Input: part model. Units: mm. Frame: model coordinates. Round coordinates to 2 decimals unless told otherwise and drop trailing zeros. Write each loop counter-clockwise with the first axis right and the second up, starting at its lowest first coordinate (ties: lowest second). Pieces come first, ordered by that corner, then holes. Notation, with made-up numbers: (-35.5, -15) - (-10.5, -15) arc R9 ccw to (-10.5, -7) - close; hole circle Ø6 at (46, 11.25). An arc over 180 degrees is marked (long way). Use one line per item in the form item = value.
```python
from build123d import *

# Parameters (mm, degrees)
SKETCH_1_W          = 101
SKETCH_1_H          = 19
SKETCH_1_R          = 2.025
EXTRUDE_1_DEPTH     = 2
CUT_EXTRUDE_1_DEPTH = 2
FILLET_1_R          = 1
FILLET_2_R          = 1


with BuildPart() as part:
    # 草图1 → 凸台-拉伸1 (new body)
    with BuildSketch(Plane.XY):
        Rectangle(SKETCH_1_W, SKETCH_1_H)
        with Locations((-46, 5)):
            Circle(SKETCH_1_R, mode=Mode.SUBTRACT)
        with Locations((46, 5)):
            Circle(SKETCH_1_R, mode=Mode.SUBTRACT)
        with Locations((46, -5)):
            Circle(SKETCH_1_R, mode=Mode.SUBTRACT)
        with Locations((-46, -5)):
            Circle(SKETCH_1_R, mode=Mode.SUBTRACT)
    extrude(amount=EXTRUDE_1_DEPTH)

    # 草图2 → 切除-拉伸1 (cut)
    with BuildSketch(Plane.XY.offset(2)):
        Polygon((-42, 6.5), (-42, -6.5), (-29, 6.5), align=None)
        Polygon((-24.050252532, 6.5), (-37.050252532, -6.5), (-24.050252532, -6.5), align=None)
        Polygon((-2.5, -6.5), (-2.5, 6.5), (-15.5, -6.5), align=None)
        Polygon((-7.449747468, 6.5), (-20.449747468, 6.5), (-20.449747468, -6.5), align=None)
        Polygon((42, -6.5), (29, 6.5), (42, 6.5), align=None)
        Polygon((37.050252532, -6.5), (24.050252532, -6.5), (24.050252532, 6.5), align=None)
        Polygon((20.449747468, -6.5), (7.449747468, 6.5), (20.449747468, 6.5), align=None)
        Polygon((15.5, -6.5), (2.5, -6.5), (2.5, 6.5), align=None)
    extrude(amount=-CUT_EXTRUDE_1_DEPTH, mode=Mode.SUBTRACT)

    # 圆角1
    fillet_1_edges = [part.edges().sort_by_distance(p)[0] for p in [
        (-20.449747468, -6.5, 1),
        (-20.449747468, 6.5, 1),
        (-7.449747468, 6.5, 1),
        (-15.5, -6.5, 1),
        (-2.5, 6.5, 1),
        (-2.5, -6.5, 1),
        (42, 6.5, 1),
        (42, -6.5, 1),
        (29, 6.5, 1),
        (-24.050252532, 6.5, 1),
        (-24.050252532, -6.5, 1),
        (-37.050252532, -6.5, 1),
        (2.5, 6.5, 1),
        (15.5, -6.5, 1),
        (2.5, -6.5, 1),
        (20.449747468, 6.5, 1),
        (20.449747468, -6.5, 1),
        (7.449747468, 6.5, 1),
        (24.050252532, 6.5, 1),
        (37.050252532, -6.5, 1),
        (24.050252532, -6.5, 1),
        (-42, 6.5, 1),
        (-29, 6.5, 1),
        (-42, -6.5, 1),
    ]]
    fillet(fillet_1_edges, radius=FILLET_1_R)

    # 圆角2
    fillet_2_edges = [part.edges().sort_by_distance(p)[0] for p in [
        (-50.5, 9.5, 1),
        (50.5, 9.5, 1),
        (50.5, -9.5, 1),
        (-50.5, -9.5, 1),
    ]]
    fillet(fillet_2_edges, radius=FILLET_2_R)


solid = part.part
```
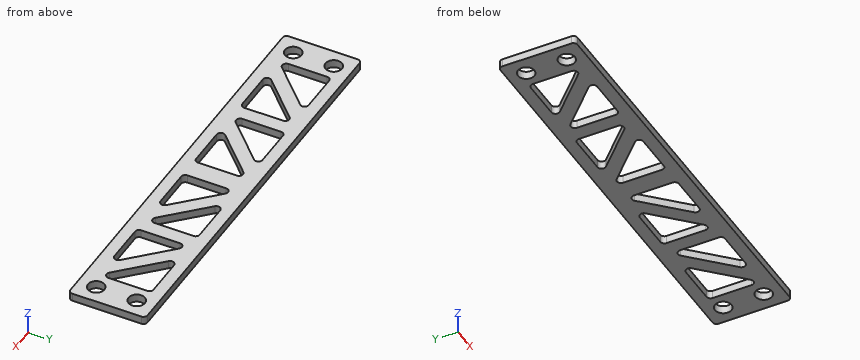
(1) Material intervals for L1, parallel to Y at x = 46, z = 0.6 (3 decimals); L2, parallel to Y at x = 9, z = 1.5; L3, parallel to X at y = 6.75, z = 0.5, sorted ascending.
Derived:
L1 = -9.5 to -7.025, -2.975 to 2.975, 7.025 to 9.5
L2 = -9.5 to -6.5, 0 to 5, 6 to 9.5
L3 = -50.5 to -47.02, -44.98 to 44.98, 47.02 to 50.5
(2) Cut plane B-B on z = 1.25. Count the separate pieces of the cut face and the enclosed holes in it, then the cut area to 3 significant figures.
Derived:
separate_pieces = 1
enclosed_holes = 12
area = 1,210 mm^2
(3) First-contact query: pin 1 Ø5 at (x, y) = (25.5, 5.5) entering from -Z; pin 2 Ø2.5 at (x, y) = (-46, 5) entering from -Z. Flat tips, straight axial feed; report the tip coordinate or a pass-through.
Derived:
pin_1 = 0
pin_2 = through
(4) Cut plane A-A on x = -46. Output: boundary loops of the cut face in (y, z) (3 decimals), then the cut area to 3 significant figures.
Derived:
outline = (-9.5, 0) - (-7.025, 0) - (-7.025, 2) - (-9.5, 2) - close; (-2.975, 0) - (2.975, 0) - (2.975, 2) - (-2.975, 2) - close; (7.025, 0) - (9.5, 0) - (9.5, 2) - (7.025, 2) - close
area = 21.8 mm^2
